Build history of the part. All positions in model axes, mm. Face numbers are marked on the shaded views. Give positions to 0.01 mm unless a question says otherwise; leave off trailing zeros. Loops run counter-clockwise (first coordinate to the right, second up) from the corner with the lowest first, then second, coordinate; pieces in that order, holes last. Notation, with made-up numbers: (48.5, -30.75) -> (88.5, -30.75) arc R22 ccw to (88.5, 2.25) -> close; hole circle Ø4 at (82.5, 86). An arc over 180 degrees is marked (long way). Answer in a Markdown table with one row per item. Add a question column.
from build123d import *
from OCP.BRepFilletAPI import BRepFilletAPI_MakeChamfer

# Parameters (mm, degrees)
EXTRUSION1_DEPTH = 15
CHANFREIN1_SIZE  = 1
CHANFREIN1_SIZE2 = 0.577350269


with BuildPart() as part:
    # Esquisse1 → Extrusion1 (new body)
    with BuildSketch(Plane.XY):
        with BuildLine():
            Line((-2, 14.866068747), (-2, 13.351029923))
            ThreePointArc((-2, 13.351029923), (0, -13.5), (2, 13.351029923))
            Line((2, 13.351029923), (2, 14.866068747))
            ThreePointArc((2, 14.866068747), (0, -15), (-2, 14.866068747))
        make_face()
    extrude(amount=EXTRUSION1_DEPTH)

    # Chanfrein1: one chamfer whose edges measure the first distance from different faces: ONE call of the kernel's chamfer builder (chamfer() names one face for all edges)
    chanfrein1_edges_1 = [part.edges().sort_by_distance(p)[0] for p in [
        (0, -15, 15),
    ]]
    chanfrein1_side_1 = [part.faces().sort_by_distance(p)[0] for p in [
        (0, -15, 7.5),
    ]]
    chanfrein1_edges_2 = [part.edges().sort_by_distance(p)[0] for p in [
        (0, -15, 0),
    ]]
    chanfrein1_side_2 = [part.faces().sort_by_distance(p)[0] for p in [
        (2.423318091, 14.108549335, 0),
    ]]
    chanfrein1 = BRepFilletAPI_MakeChamfer(part.part.solid().wrapped)
    for e in chanfrein1_edges_1:
        chanfrein1.Add(CHANFREIN1_SIZE, CHANFREIN1_SIZE2, e.wrapped, chanfrein1_side_1[0].wrapped)  # the first distance lies on this face
    for e in chanfrein1_edges_2:
        chanfrein1.Add(CHANFREIN1_SIZE, CHANFREIN1_SIZE2, e.wrapped, chanfrein1_side_2[0].wrapped)  # the first distance lies on this face
    add(Compound.cast(chanfrein1.Shape()), mode=Mode.REPLACE)


solid = part.part
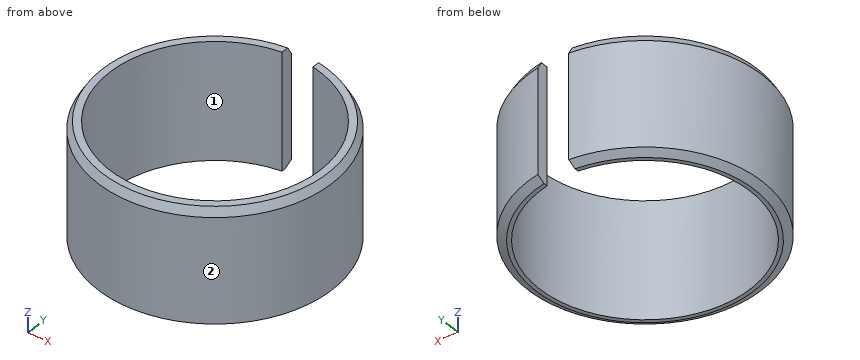
(1) Saw through at C-C, the plane z = 6.5. List the corners of the cut face in (x, y).
(2) Two-plate mould, pull along Y, no slides. Class the marked faces 1 and 2: released by +Y, released by -Y, zero draft, split by the parting line, or undercut.
(3) Saw through at A-A, the plane y = 0. List the corners of the cut face in (x, z).
(4) Flat gauge pins, fed straight in: pin 1 Ø5 at (x, y) = (2, -9.5) entering from +Z; pin 2 Ø1.7 at (y, z) = (14, 4.5) entering from +X; pin 3 Ø1.7 at (y, z) = (14, 6) entering from -X; pin 4 Ø1.5 at (x, z) = (12, 11) entering from -Y. Where does each tip first touch, or does it go through?
(5) Wall check: line 1 along X through (y, z) = (0.25, 2.75); line 2 along X through (y, z) = (10.5, 9.75); line 3 along Y through (x, z) = (-11.25, 10). Give the ranges that are in metal, low to high. Write a range as from..to.
(6) Saw through at B-B, the plane x = 0. List the corners of the cut face in (y, z), then the cut area to 3 significant figures.
Worked answers:
| question | item | result |
|---|---|---|
| 1 | outline | (-2, 13.35) -> (-2, 14.87) arc R15 ccw (long way) to (2, 14.87) -> (2, 13.35) arc R13.5 cw (long way) to start |
| 2 | face 1 | undercut |
| 2 | face 2 | split by the parting line |
| 3 | outline | (-15, 0.58) -> (-14, 0) -> (-13.5, 0) -> (-13.5, 15) -> (-14.42, 15) -> (-15, 14) -> close; (13.5, 0) -> (14, 0) -> (15, 0.58) -> (15, 14) -> (14.42, 15) -> (13.5, 15) -> close |
| 4 | pin 1 | through |
| 4 | pin 2 | x = 7.22 |
| 4 | pin 3 | x = -7.22 |
| 4 | pin 4 | y = -9.92 |
| 5 | line 1 | -15..-13.5, 13.5..15 |
| 5 | line 2 | -10.71..-8.49, 8.49..10.71 |
| 5 | line 3 | -9.92..-7.46, 7.46..9.92 |
| 6 | outline | (-15, 0.58) -> (-14, 0) -> (-13.5, 0) -> (-13.5, 15) -> (-14.42, 15) -> (-15, 14) -> close |
| 6 | area | 21.9 mm^2 |
